from build123d import *

# Parameters (mm, degrees)
F0_R     = 2
F0_R_2   = 1.75
F1_DEPTH = 4
F2_DEPTH = 2


with BuildPart() as f1:
    # F0 (on Top) → F1 (new body)
    with BuildSketch(Plane.XY):
        with BuildLine():
            Line((2, 0), (2, 1.0307764064))
            ThreePointArc((2, 1.0307764064), (-2.25, 0), (2, -1.0307764064))
            Line((2, -1.0307764064), (2, 0))
        make_face()
        Circle(F0_R, mode=Mode.SUBTRACT)
        Circle(F0_R)
        Circle(F0_R_2, mode=Mode.SUBTRACT)
    extrude(amount=F1_DEPTH)

    # F0 (on Top) → F2 (join)
    with BuildSketch(Plane.XY):
        Circle(F0_R)
        Circle(F0_R_2, mode=Mode.SUBTRACT)
    extrude(amount=-F2_DEPTH)


solid = f1.part
Read the model definition and answer for the solid it produces. Units are mm, in the model's axes. A direction names the side the tool comes from. Coordinates: 2 decimals unless noted, no trailing zeros. Order: outer loops, then holes, each group sorted by start corner. A loop starts at its lowest first (then second) coordinate and runs counter-clockwise, first axis right, second up. Notation, with made-up numbers: (-2, 25.25) -> (18, 25.25) arc R14 cw to (18, 32.25) -> close; hole circle Ø10 at (44, -13.5). An arc over 180 degrees is marked (long way). Answer as a JSON object with one key per item and string values.
1) Consider line 1 along Y through (x, z) = (0, -1.1); line 2 along Y through (x, z) = (0, 1.3); line 3 along X through (y, z) = (1, -0.2). Determine where each line is inside the solid, lowest interval first. Write a range as from..to.
Model answer:
{"line 1": "y = -2..-1.75, 1.75..2", "line 2": "y = -2.25..-1.75, 1.75..2.25", "line 3": "x = -1.73..-1.44, 1.44..1.73"}
2) A cutting plane is placed at A-A, the plane x = 0. Determine the outline of the cut face in (y, z).
Model answer:
{"outline": "(-2.25, 0) -> (-2, 0) -> (-2, -2) -> (-1.75, -2) -> (-1.75, 4) -> (-2.25, 4) -> close; (1.75, -2) -> (2, -2) -> (2, 0) -> (2.25, 0) -> (2.25, 4) -> (1.75, 4) -> close"}
3) A tool of negligible diameter and unlimited length cuts with its end or side. For faces 1 (the face through (0, -2, -1)), 2 (the face through (2, 0, 2)), from which of +Z, -Z, +X, -X, +Y, -Y can it reach the whole face along a straight path? Write none if from no direction.
Model answer:
{"face 1": "-Z", "face 2": "+Z, -Z, +X, +Y, -Y"}
4) A cutting plane is placed at C-C, the plane z = 0.5. Determine the outline of the cut face in (x, y), plus the area to 3 significant figures.
Model answer:
{"outline": "(2, -1.03) -> (2, 1.03) arc R2.25 ccw (long way) to start; hole circle Ø3.5 at (0, 0)", "area": "5.94 mm²"}
5) A cutting plane is placed at B-B, the plane y = -0.8. Determine the outline of the cut face in (x, z).
Model answer:
{"outline": "(-2.1, 0) -> (-1.83, 0) -> (-1.83, -2) -> (-1.56, -2) -> (-1.56, 4) -> (-2.1, 4) -> close; (1.56, -2) -> (1.83, -2) -> (1.83, 0) -> (2, 0) -> (2, 4) -> (1.56, 4) -> close"}
6) Each of these flat-tipped pins is pushed along its axis until it touches: pin 1 (1 mm diameter, centred on y = 1, z = 1, fed in from -X); pin 2 (1.5 mm diameter, centred on x = -2, z = 2, fed in from -Y). Where does it stop, or does it pass through?
Model answer:
{"pin 1": "stops at x = -2.19", "pin 2": "stops at y = -1.87"}
7) A cutting plane is placed at D-D, the plane z = -0.2. Determine the outline of the cut face in (x, y), plus the area to 3 significant figures.
Model answer:
{"outline": "circle Ø4 at (0, 0); hole circle Ø3.5 at (0, 0)", "area": "2.95 mm²"}
